```python
from build123d import *

# Parameters (mm, degrees)
SKETCH1_R           = 1.5
BOSS_EXTRUDE1_DEPTH = 6.9
CUT_EXTRUDE2_DEPTH  = 4.9
SKETCH5_R           = 1
CUT_EXTRUDE3_DEPTH  = 14
SKETCH8_R           = 1
CUT_EXTRUDE5_DEPTH  = 17


with BuildPart() as part:
    # Sketch1 → Boss-Extrude1 (new body)
    with BuildSketch(Plane.XY):
        with BuildLine():
            Line((9.631516349, 18.000341084), (29.676516349, 18.000341084))
            ThreePointArc((29.676516349, 18.000341084), (36.383041872, 11.97511352), (31.10792826, 4.663887347))
            Line((31.10792826, 4.663887347), (9.631516349, 0))
            Line((9.631516349, 0), (9.631516349, 4))
            Line((9.631516349, 4), (4, 4))
            Line((4, 4), (4, 0))
            Line((4, 0), (0, 0))
            Line((0, 0), (0, 18.000341084))
            Line((0, 18.000341084), (4, 18.000341084))
            Line((4, 18.000341084), (4, 14.000341084))
            Line((4, 14.000341084), (9.631516349, 14.000341084))
            Line((9.631516349, 14.000341084), (9.631516349, 18.000341084))
        make_face()
        with Locations((29.676516349, 11.255296941)):
            Circle(SKETCH1_R, mode=Mode.SUBTRACT)
    extrude(amount=BOSS_EXTRUDE1_DEPTH)

    # Sketch4 → Cut-Extrude2 (cut)
    with BuildSketch(Plane.XY):
        with BuildLine():
            Line((21.876472206, 2.659154375), (21.876472206, 18.000341084))
            Line((21.876472206, 18.000341084), (29.676516349, 18.000341084))
            ThreePointArc((29.676516349, 18.000341084), (36.383041872, 11.97511352), (31.10792826, 4.663887347))
            Line((31.10792826, 4.663887347), (31.10792826, 2.659154375))
            Line((31.10792826, 2.659154375), (21.876472206, 2.659154375))
        make_face()
    extrude(amount=CUT_EXTRUDE2_DEPTH, mode=Mode.SUBTRACT)

    # Sketch5 → Cut-Extrude3 (cut)
    with BuildSketch(Plane.ZY):
        with Locations((2.45, 8)):
            Circle(SKETCH5_R)
    extrude(amount=-CUT_EXTRUDE3_DEPTH, mode=Mode.SUBTRACT)

    # Sketch8 → Cut-Extrude5 (cut)
    with BuildSketch(Plane(origin=(19.746237848, -5.290988485, 0), x_dir=(0, 0, -1), z_dir=(0.965925826, -0.258819045, 0))):
        with Locations((-2.45, 11.2)):
            Circle(SKETCH8_R)
    extrude(amount=-CUT_EXTRUDE5_DEPTH, mode=Mode.SUBTRACT)


solid = part.part
```
Read the model definition and answer for the solid it produces. Units are mm, in the model's axes. A direction names the side the tool comes from. Give positions to 0.01 mm unless a question says otherwise; leave off trailing zeros. Loops run counter-clockwise (first coordinate to the right, second up) from the corner with the lowest first, then second, coordinate; pieces in that order, holes last.
Item 1: The part is cut by section A-A (x = 3). Write down the section's boundary in (y, z).
Item 2: The part is cut by section B-B (y = 12). Write down the section's boundary in (x, z), and give its area (3 significant figures).
Item 3: For faces 4 (the flat face through (4, 16, 3)), 5 (the flat face through (28, 10, 4.9)), 6 (the cylindrical face through (6.615, 7.024, 2.233)), 7 (the flat face through (7, 4, 3)), determine the directions among +Z, -Z, +X, -X, +Y, -Y from which every point of the face is accessible in a straight line to the end or side of a thin tool.
Item 4: Each of these flat-tipped pins is pushed along its axis until it touches: pin 1 Ø5 at (x, y) = (32.5, 10.5) entering from -Z; pin 2 Ø2.5 at (x, y) = (29.68, 11.26) entering from +Z; pin 3 Ø4 at (y, z) = (9, 3) entering from +X; pin 4 Ø1.2 at (y, z) = (15.5, 2) entering from +X. Where does it stop, or does it pass through?
Item 5: The mould has two halves that part along X. Classify faces 1 (the flat face through (2, 18, 3)), 2 (the cylindrical face through (36.367, 12.112, 5.886)), 3 (the flat face through (7, 14, 3)): released by +X, released by -X, zero draft, split by the parting line, or undercut.
Item 6: Find the intervals of material crossed by line 1 along Y through (x, z) = (4.5, 2.45); line 2 along Y through (x, z) = (6, 5); line 3 along X through (y, z) = (13.75, 4.75), in increasing order.
Item 7: The part is cut by section D-D (y = 3). Write down the section's boundary in (x, z).
Item 8: The part is cut by section C-C (z = 3). Write down the section's boundary in (x, y).
Taken from the geometry:
1. outline: (0, 0) - (18, 0) - (18, 6.9) - (0, 6.9) - close; hole circle Ø2 at (8, 2.45)
2. outline: (0, 0) - (21.88, 0) - (21.88, 4.9) - (28.37, 4.9) - (28.37, 6.9) - (0, 6.9) - close; (30.98, 4.9) - (36.38, 4.9) - (36.38, 6.9) - (30.98, 6.9) - close
2. area: 175 mm2
3. face 4: +Z, -Z, +Y
3. face 5: -Z, +X, +Y, -Y
3. face 6: -X
3. face 7: +Z, -Z, -Y
4. pin 1: stops at z = 4.9
4. pin 2: passes through
4. pin 3: stops at x = 36.22
4. pin 4: stops at x = 21.88
5. face 1: zero draft
5. face 2: released by +X
5. face 3: undercut
6. line 1: y = 4 to 7, 9 to 14
6. line 2: y = 4 to 14
6. line 3: x = 0 to 21.88
7. outline: (0, 0) - (4, 0) - (4, 6.9) - (0, 6.9) - close; (9.63, 0) - (21.88, 0) - (21.88, 4.9) - (23.45, 4.9) - (23.45, 6.9) - (9.63, 6.9) - close
8. outline: (0, 0) - (4, 0) - (4, 4) - (9.63, 4) - (9.63, 0) - (21.88, 2.66) - (21.88, 4.87) - (13.31, 7.16) - (0, 7.16) - close; (0, 8.84) - (7.07, 8.84) - (6.01, 9.12) - (6.44, 10.73) - (13.53, 8.84) - (14, 8.84) - (14, 8.71) - (21.88, 6.6) - (21.88, 18) - (9.63, 18) - (9.63, 14) - (4, 14) - (4, 18) - (0, 18) - close
